Can you work these out from the model? Positions are in its coordinate system, mm. Round coordinates to 2 decimals unless told otherwise and drop trailing zeros. Order: outer loops, then holes, each group sorted by start corner. A loop starts at its lowest first (then second) coordinate and runs counter-clockwise, first axis right, second up. Notation, with made-up numbers: M -8,50.5 L 49,50.5 A5 cw 49,55.5 Z; hole C -33.5,6.5 d5. An arc over 180 degrees is marked long. Answer as a JSON object with one key per item and string values. Group by question number.
from build123d import *

# Parameters (mm, degrees)
F0_R     = 7.5
F2_DEPTH = 50


with BuildPart() as f2:
    # F0 (on Front) → F2 (new body)
    with BuildSketch(Plane.XZ):
        with BuildLine():
            ThreePointArc((-20.2771231268, 72.2069129495), (-35.691129754, 80.8618774554), (-27.0361647105, 96.2758837807))
            ThreePointArc((-27.0361647105, 96.2758837807), (-83.9922641187, 54.2706142236), (-98.8813425816, -14.9157664658))
            ThreePointArc((-98.8813425816, -14.9157664658), (-88.3856453807, -0.6911276961), (-74.161006875, -11.1868252548))
            ThreePointArc((-74.161006875, -11.1868252548), (-62.9941980859, 40.7029606726), (-20.2771231268, 72.2069129495))
        make_face()
        with BuildLine():
            ThreePointArc((-11.1566443384, 84.2413982472), (-16.1066113799, 94.2036772197), (-27.0361647105, 96.2758837807))
            ThreePointArc((-27.0361647105, 96.2758837807), (-35.691129754, 80.8618774554), (-20.2771231268, 72.2069129495))
            ThreePointArc((-20.2771231268, 72.2069129495), (-13.6943651026, 76.6913656362), (-11.1566443384, 84.2413982472))
        make_face()
        with Locations((-23.6566443384, 84.2413982472)):
            Circle(F0_R, mode=Mode.SUBTRACT)
        with BuildLine():
            ThreePointArc((-74.161006875, -11.1868252548), (-88.3856453807, -0.6911276961), (-98.8813425816, -14.9157664658))
            ThreePointArc((-98.8813425816, -14.9157664658), (-85.5863211984, -25.5162884811), (-74.0211747752, -13.0512955493))
            ThreePointArc((-74.0211747752, -13.0512955493), (-74.0561818199, -12.1164422861), (-74.161006875, -11.1868252548))
        make_face()
        with Locations((-86.5211747752, -13.0512955493)):
            Circle(F0_R, mode=Mode.SUBTRACT)
        with Locations((-23.6566443384, 84.2413982472)):
            Circle(F0_R)
        with Locations((-86.5211747752, -13.0512955493)):
            Circle(F0_R)
    extrude(amount=F2_DEPTH)


solid = f2.part
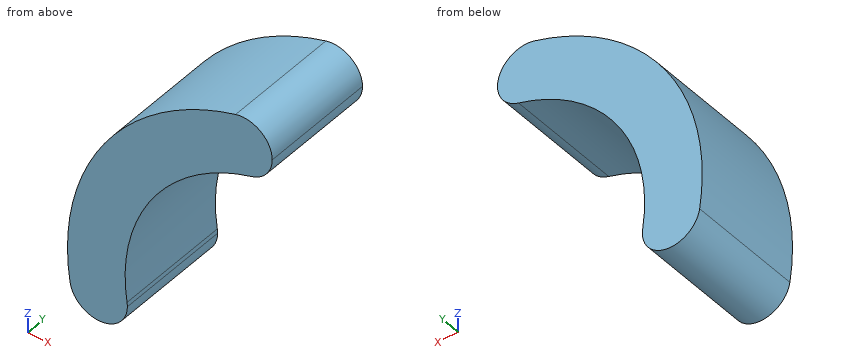
Item 1: Suppose I cut it at A-A, the plane y = -19. Write out the boundary of the cut face in (x, z), and give its area (3 significant figures).
Item 2: Suppose I cut it at B-B, the plane z = 56. Write out the boundary of the cut face in (x, y).
Item 3: I need wall thicknesses on line 1 (X direction, y = -23, z = 51); line 2 (Z direction, x = -89.5, y = -46.5); line 3 (Z direction, x = -46, y = -41.5). Which ranges of each line are inside material? Lowest first, please.
Item 4: Suppose I cut it at C-C, the plane x = -29. Write out the boundary of the cut face in (y, z).
Item 5: I'm going to push flat-ended pins straight in: pin 1 Ø12 at (x, y) = (-28.5, -16) entering from -Z; pin 2 Ø4 at (x, y) = (-34, -44) entering from +Z; pin 3 Ø8 at (x, y) = (-32.5, -6.5) entering from -Z. Where does each tip first touch, or does it pass through?
Computed:
{
 "1": {"outline": "M -98.88,-14.92 A12.5 ccw -74.16,-11.19 A75 cw -20.28,72.21 A12.5 ccw -27.04,96.28 A100 ccw Z", "area": "3,660 mm^2"},
 "2": {"outline": "M -82.85,-50 L -49.89,-50 L -49.89,0 L -82.85,0 Z"},
 "3": {"line 1": "x = -86.02 to -54.99", "line 2": "z = -25.19 to 44.61", "line 3": "z = 59.24 to 88.79"},
 "4": {"outline": "M -50,69.17 L 0,69.17 L 0,95.7 L -50,95.7 Z"},
 "5": {"pin 1": "stops at z = 66.59", "pin 2": "stops at z = 94.74", "pin 3": "stops at z = 65.52"}
}
